Read the model definition and answer for the solid it produces. Units are mm, in the model's axes. A direction names the side the tool comes from. Coordinates: 2 decimals unless noted, no trailing zeros. Loops run counter-clockwise (first coordinate to the right, second up) from the corner with the lowest first, then second, coordinate; pieces in that order, holes last.
from build123d import *

# Parameters (mm, degrees)
SKETCH_1_W          = 5
SKETCH_1_H          = 10
EXTRUDE_1_DEPTH     = 8
CUT_EXTRUDE_1_DEPTH = 8
EXTRUDE_2_DEPTH     = 5
SKETCH_5_W          = 4
SKETCH_5_H          = 2.5
CUT_EXTRUDE_2_DEPTH = 5
SKETCH_4_W          = 1.118033989
SKETCH_4_H          = 4
CUT_EXTRUDE_3_DEPTH = 5
SKETCH_8_W          = 4
SKETCH_8_H          = 1.4
CUT_EXTRUDE_4_DEPTH = 1.8
SKETCH_10_W         = 1.8
SKETCH_10_H         = 4
CUT_EXTRUDE_5_DEPTH = 2
SKETCH_11_R         = 0.25
CUT_EXTRUDE_6_DEPTH = 10


with BuildPart() as part:
    # 草图1 → 凸台-拉伸1 (new body)
    with BuildSketch(Plane(origin=(0, 0, 0), x_dir=(0, 0, -1), z_dir=(1, 0, 0))):
        Rectangle(SKETCH_1_W, SKETCH_1_H)
    extrude(amount=EXTRUDE_1_DEPTH)

    # 草图2 → 切除-拉伸1 (cut)
    with BuildSketch(Plane.XY.offset(2.5)):
        Polygon((8, 5), (1, 5), (1, -0.636116149), (2.8, -1.507895938), (2.8, -2.907895938), (0.7, -4.264361935), (0, -4.264361935), (0, -5), (8, -5), align=None)
    extrude(amount=-CUT_EXTRUDE_1_DEPTH, mode=Mode.SUBTRACT)

    # 草图3 → 凸台-拉伸2 (add)
    with BuildSketch(Plane.XY.offset(2.5)):
        Polygon((1, 5), (1, 5.5), (0, 5), align=None)
    extrude(amount=-EXTRUDE_2_DEPTH)

    # 草图5 → 切除-拉伸2 (cut)
    with BuildSketch(Plane.ZY):
        with Locations((0, 3.75)):
            Rectangle(SKETCH_5_W, SKETCH_5_H)
    extrude(amount=-CUT_EXTRUDE_2_DEPTH, mode=Mode.SUBTRACT)

    # 草图4 → 切除-拉伸3 (cut)
    with BuildSketch(Plane(origin=(-2, 4, 0), x_dir=(0.8944271909999156, 0.44721359549995865, 0), z_dir=(-0.44721359549995865, 0.8944271909999156, 0))):
        with Locations((2.795084972, 0)):
            Rectangle(SKETCH_4_W, SKETCH_4_H)
    extrude(amount=-CUT_EXTRUDE_3_DEPTH, mode=Mode.SUBTRACT)

    # 草图8 → 切除-拉伸4 (cut)
    with BuildSketch(Plane(origin=(2.8, 0, 0), x_dir=(0, 0, -1), z_dir=(1, 0, 0))):
        with Locations((0, -2.207895938)):
            Rectangle(SKETCH_8_W, SKETCH_8_H)
    extrude(amount=-CUT_EXTRUDE_4_DEPTH, mode=Mode.SUBTRACT)

    # 草图10 → 切除-拉伸5 (cut)
    with BuildSketch(Plane.XZ.offset(1.507895938)):
        with Locations((1.9, 0)):
            Rectangle(SKETCH_10_W, SKETCH_10_H)
    extrude(amount=-CUT_EXTRUDE_5_DEPTH, mode=Mode.SUBTRACT)

    # 草图11 → 切除-拉伸6 (cut)
    with BuildSketch(Plane(origin=(0, 0, -2.5), x_dir=(-1, 0, 0), z_dir=(0, 0, -1))):
        with Locations((-0.5, 4.55)):
            Circle(SKETCH_11_R)
    extrude(amount=-CUT_EXTRUDE_6_DEPTH, mode=Mode.SUBTRACT)


solid = part.part
Item 1: A cutting plane is placed at D-D on x = 2.3. Determine the outline of the cut face in (y, z), then the cut area to 3 significant figures.
Numbers:
outline: (-3.23, -2.5) - (-1.27, -2.5) - (-1.27, -2) - (-2.91, -2) - (-2.91, 2) - (-1.27, 2) - (-1.27, 2.5) - (-3.23, 2.5) - close
area: 3.26 mm2
Item 2: A cutting plane is placed at A-A on x = 0.5. Determine the outline of the cut face in (y, z), then the cut area to 3 significant figures.
Numbers:
outline: (-4.26, -2.5) - (4.3, -2.5) - (4.3, -2) - (2.5, -2) - (2.5, 2) - (4.3, 2) - (4.3, 2.5) - (-4.26, 2.5) - close; (4.8, -2.5) - (5.25, -2.5) - (5.25, -2) - (4.8, -2) - close; (4.8, 2) - (5.25, 2) - (5.25, 2.5) - (4.8, 2.5) - close
area: 36.1 mm2
Item 3: Which of the six approach directions +Z, -Z, +X, -X, +Y, -Y give full straight-line access (tool end or side, diameter ignored) to faces 4 (the face through (0.8, -0.4, -2.5)), 5 (the face through (2, -2.908, 0)), 6 (the face through (0.5, 3.6, -2))?
Numbers:
face 4: -Z, +X, -X, +Y, -Y
face 5: +X, +Y
face 6: +X, -X, +Y
Item 4: A cutting plane is placed at C-C on z = -1.35. Determine the outline of the cut face in (x, y), then the cut area to 3 significant figures.
Numbers:
outline: (0, -4.26) - (0.7, -4.26) - (2.8, -2.91) - (1, -2.91) - (1, 2.5) - (0, 2.5) - close
area: 7.78 mm2
Item 5: A cutting plane is placed at B-B on y = 4.55. Determine the outline of the cut face in (x, z).
Numbers:
outline: (0, -2.5) - (0.25, -2.5) - (0.25, -2) - (0, -2) - close; (0, 2) - (0.25, 2) - (0.25, 2.5) - (0, 2.5) - close; (0.75, -2.5) - (1, -2.5) - (1, -2) - (0.75, -2) - close; (0.75, 2) - (1, 2) - (1, 2.5) - (0.75, 2.5) - close
Item 6: Find the intervals of material crossed by line 1 along Y through (x, z) = (0.4, 0.6); line 2 along X through (y, z) = (-0.5, -1.6); line 3 along Z through (x, y) = (0.7, 4.25), in increasing order.
Numbers:
line 1: y = -4.26 to 2.5
line 2: x = 0 to 1
line 3: z = -2.5 to -2, 2 to 2.5
Item 7: Given pin 1 (1.5 mm diameter, centred on x = 2, z = -1.5, fed in from +Y); pin 2 (0.8 mm diameter, centred on x = 0.5, z = 0, fed in from +Y), each flat-ended and moving along its own axis, determine where each tip first touches the part or whether it passes through.
Numbers:
pin 1: stops at y = -0.85
pin 2: stops at y = 2.5
Item 8: Determine the mould class of faces 1 (the face through (1.887, -1.066, -2.246)), 2 (the face through (0.8, -0.4, 2.5)), 3 (the face through (2, -2, 2)) for opening direction Z: released by +Z, released by -Z, zero draft, split by the parting line, or undercut.
Numbers:
face 1: zero draft
face 2: released by +Z
face 3: undercut
